Autodesk Inventor part; units mm, degrees
ref_plane "YZ Plane" through (0, 0, 0) normal (1, 0, 0) x (0, 1, 0)
ref_plane "XZ Plane" through (0, 0, 0) normal (0, 1, 0) x (-1, 0, 0)
ref_plane "XY Plane" through (0, 0, 0) normal (0, 0, 1) x (1, 0, 0)
sketch "Sketch1" plane through (0, 0, 0) normal (0, 0, 1) x (1, 0, 0)
  line L0 (0, 158.9) -> (0, -158.9) construction
  line L1 (-125.3, 0) -> (125.3, 0) construction
  line L2 (89.5, -113.5) -> (-89.5, -113.5)
  line L3 (-89.5, -113.5) -> (-89.5, 113.5)
  line L4 (-89.5, 113.5) -> (89.5, 113.5)
  line L5 (89.5, 113.5) -> (89.5, -113.5)
  line L6 (89.5, -113.5) -> (-89.5, 113.5) construction
  line L7 (-89.5, -113.5) -> (89.5, 113.5) construction
  point P0 (0, 0)
  dimension "d4" = 227
  dimension "d5" = 179
extrude "Extrusion3" add sketch "Sketch1" along normal mid plane 412
sketch "Sketch2" plane through (-89.5, -113.5, 206) normal (0, -1, 0) x (1, 0, 0)
  line L0 (179, -412) -> (179, 0)
  line L1 (0, 0) -> (179, 0)
  line L2 (0, 0) -> (0, -412)
  line L3 (179, -412) -> (0, -412)
  line L4 (109.5, -16) -> (10, -16)
  line L5 (10, -16) -> (10, -396)
  line L6 (10, -396) -> (109.5, -396)
  line L7 (109.5, -396) -> (109.5, -16)
  line L8 (109.5, -16) -> (10, -396) construction
  line L9 (10, -16) -> (109.5, -396) construction
  line L10 (169, -96) -> (109.5, -96)
  line L11 (109.5, -96) -> (109.5, -316)
  line L12 (109.5, -316) -> (169, -316)
  line L13 (169, -316) -> (169, -96)
  line L14 (169, -96) -> (109.5, -316) construction
  line L15 (109.5, -96) -> (169, -316) construction
  point P0 (89.5, -206)
  point P1 (59.75, -206)
  point P2 (139.25, -206)
  point P3 (59.75, -206)
  point P4 (139.25, -206)
  dimension "d8" = 220
  dimension "d9" = 380
  dimension "d10" = 10
  dimension "d11" = 10
  dimension "d12" = 20
extrude "Extrusion4" cut sketch "Sketch2" against normal blind 28.5
sketch "Sketch3" plane through (-89.5, -85, 206) normal (0, -1, 0) x (1, 0, 0)
  circle A0 centre (129.1, -361.5) radius 16.2143
  circle A1 centre (129.1, -50.5) radius 16.2143
  line L0 (179, -412) -> (0, -412)
  line L1 (0, 0) -> (179, 0)
  line L2 (89.5, 82.4) -> (89.5, -494.4)
  point P0 (89.5, -206)
  dimension "d17" = 311
  dimension "d18" = 50.5
  dimension "d20" = 50.5
  dimension "d21" = 39.6
extrude "Extrusion5" add sketch "Sketch3" along normal blind 10.5
sketch "Sketch4" plane through (39.6, -95.5, -155.5) normal (0, -1, 0) x (1, 0, 0)
  circle A0 centre (0, 0) radius 16.2143
  circle A1 centre (0, 311) radius 16.2143
  line L0 (49.9, 361.5) -> (49.9, -50.5)
  line L1 (-129.1, 361.5) -> (49.9, 361.5)
  line L2 (-129.1, -50.5) -> (-129.1, 361.5)
  line L3 (49.9, -50.5) -> (-129.1, -50.5)
  line L4 (-19.6, 265.5) -> (-19.6, 345.5)
  line L5 (39.9, 265.5) -> (-19.6, 265.5)
  line L6 (39.9, 45.5) -> (39.9, 265.5)
  line L7 (-19.6, 45.5) -> (39.9, 45.5)
  line L8 (-19.6, -34.5) -> (-19.6, 45.5)
  line L9 (-119.1, -34.5) -> (-19.6, -34.5)
  line L10 (-119.1, 345.5) -> (-119.1, -34.5)
  line L11 (-19.6, 345.5) -> (-119.1, 345.5)
  point P0 (-39.6, 155.5)
hole "Hole1" at (39.6, -95.5, -155.5) at (39.6, -95.5, 155.5) direction (0, 1, 0) diameter 6.647 depth 10 tip angle 118
equation "\"d18\" = d20"
properties part number "17-0028-0034" material "ABS Plastic"
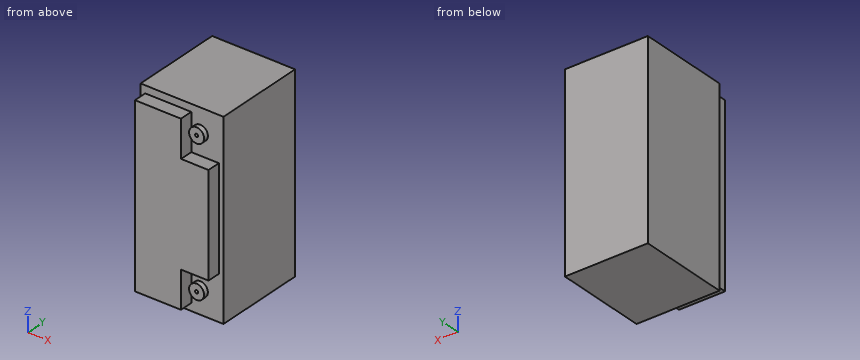
Check sheet for the modelled part. Datum: model origin and axes. Units: mm. Coordinates: 2 decimals unless noted, no trailing zeros. Loops run counter-clockwise (first coordinate to the right, second up) from the corner with the lowest first, then second, coordinate; pieces in that order, holes last. Notation, with made-up numbers: (8.5, -27) -> (39.5, -27) arc R24 cw to (39.5, -10) -> close; hole circle Ø3 at (74, 56.5). An arc over 180 degrees is marked (long way). Answer in a Markdown table with one row per item.
1. Go/stop test with flat-tipped pins: pin 1 (8.5 mm diameter, centred on y = -103, z = -158.5, fed in from +X); pin 2 (4 mm diameter, centred on x = 39.6, z = -155.5, fed in from -Y); pin 3 (6 mm diameter, centred on x = 39.6, z = 155.5, fed in from -Y). Record where each tip stops, or that it passes through.
Check values:
| item | result |
|---|---|
| pin 1 | stops at x = 20 |
| pin 2 | stops at y = -84.7 |
| pin 3 | stops at y = -85.31 |
2. Material ranges on line 1 along X through (y, z) = (-90, -155); line 2 along Z through (x, y) = (39.6, -91.5); line 3 along Y through (x, z) = (27, 166.5), recorded low to high. Write a range as [from, to].
Check values:
| item | result |
|---|---|
| line 1 | x = [-79.5, 20], [23.39, 36.31], [42.89, 55.81] |
| line 2 | z = [-171.71, -158.82], [-152.18, -139.29], [-110, 110], [139.29, 152.18], [158.82, 171.71] |
| line 3 | y = [-85, 113.5] |
3. Sectioned sample at A-A, the plane x = 69.5. Record the boundary of the cut face in (y, z), then the cut area to 3 significant figures.
Check values:
| item | result |
|---|---|
| outline | (-113.5, -110) -> (-85, -110) -> (-85, -206) -> (113.5, -206) -> (113.5, 206) -> (-85, 206) -> (-85, 110) -> (-113.5, 110) -> close |
| area | 88,100 mm2 |
4. Sectioned sample at B-B, the plane x = 29.5. Record the boundary of the cut face in (y, z), then the cut area to 3 significant figures.
Check values:
| item | result |
|---|---|
| outline | (-113.5, -110) -> (-85, -110) -> (-85, -142.82) -> (-95.5, -142.82) -> (-95.5, -168.18) -> (-85, -168.18) -> (-85, -206) -> (113.5, -206) -> (113.5, 206) -> (-85, 206) -> (-85, 168.18) -> (-95.5, 168.18) -> (-95.5, 142.82) -> (-85, 142.82) -> (-85, 110) -> (-113.5, 110) -> close |
| area | 88,600 mm2 |
